Source: CAD feature listing. Evaluate the final solid. Frame: model axes, mm. A direction names the side the tool comes from. Give positions to 0.01 mm unless a question says otherwise; leave off trailing zeros. Order: outer loops, then holes, each group sorted by start corner. A loop starts at its lowest first (then second) coordinate and runs counter-clockwise, first axis right, second up. Notation, with made-up numbers: (33, -6) -> (68, -6) arc R16 ccw to (68, 12) -> close; hole circle Ø7 at (58.5, -32.5). An arc over 180 degrees is marked (long way). Answer in a Markdown table with one row per item.
```python
from build123d import *

# Parameters (mm, degrees)
BOSS_EXTRUDE1_DEPTH = 10
SKETCH4_R           = 2.5
BOSS_EXTRUDE3_DEPTH = 2.5


with BuildPart() as part:
    # Sketch1 → Boss-Extrude1 (new body)
    with BuildSketch(Plane(origin=(0, 0, 0), x_dir=(0, 0, -1), z_dir=(1, 0, 0))):
        Polygon((0, 9.55), (1.824674268, 6.809777075), (4.775, 8.270542606), (4.985102807, 4.985102807), (8.270542606, 4.775), (6.809777075, 1.824674268), (9.55, 0), (6.809777075, -1.824674268), (8.270542606, -4.775), (4.985102807, -4.985102807), (4.775, -8.270542606), (1.824674268, -6.809777075), (0, -9.55), (-1.824674268, -6.809777075), (-4.775, -8.270542606), (-4.985102807, -4.985102807), (-8.270542606, -4.775), (-6.809777075, -1.824674268), (-9.55, 0), (-6.809777075, 1.824674268), (-8.270542606, 4.775), (-4.985102807, 4.985102807), (-4.775, 8.270542606), (-1.824674268, 6.809777075), align=None)
    boss_extrude1 = extrude(amount=-BOSS_EXTRUDE1_DEPTH)

    # Sketch4 → Boss-Extrude3 (add)
    with BuildSketch(Plane(origin=(0, 0, 0), x_dir=(0, 0, -1), z_dir=(1, 0, 0))):
        Circle(SKETCH4_R)
    boss_extrude3 = extrude(amount=BOSS_EXTRUDE3_DEPTH)

    # Mirror1: Boss-Extrude1, Boss-Extrude3 across plane
    add(boss_extrude1.mirror(Plane.ZY.offset(10)))
    add(boss_extrude3.mirror(Plane.ZY.offset(10)))


solid = part.part
```
(1) Section query A-A (x = -16.75). Return the cut outline in (y, z) (3 decimals).
A:
| item | result |
|---|---|
| outline | (-9.55, 0) -> (-6.81, -1.825) -> (-8.271, -4.775) -> (-4.985, -4.985) -> (-4.775, -8.271) -> (-1.825, -6.81) -> (0, -9.55) -> (1.825, -6.81) -> (4.775, -8.271) -> (4.985, -4.985) -> (8.271, -4.775) -> (6.81, -1.825) -> (9.55, 0) -> (6.81, 1.825) -> (8.271, 4.775) -> (4.985, 4.985) -> (4.775, 8.271) -> (1.825, 6.81) -> (0, 9.55) -> (-1.825, 6.81) -> (-4.775, 8.271) -> (-4.985, 4.985) -> (-8.271, 4.775) -> (-6.81, 1.825) -> close |
(2) Pull-direction query (Z, two-part tool) for faces 1 (the flat face through (-10.14, -7.55, -3.32)), 2 (the flat face through (-10.14, -3.28, -7.53)), 3 (the flat face through (-10.14, 6.6, 4.88)); classes: +Z half, -Z half, draft (parallel to the pull), parting line (faces both ways), or undercut.
A:
| item | result |
|---|---|
| face 1 | undercut |
| face 2 | -Z half |
| face 3 | +Z half |
(3) First-contact query: pin 1 Ø10 at (x, y) = (-6.5, 4.5) entering from -Z; pin 2 Ø3 at (x, y) = (-5.5, -5) entering from +Z; pin 3 Ø10 at (x, z) = (-2, -6) entering from -Y; pin 4 Ø5 at (y, z) = (7, 3) entering from +X. Flat tips, straight axial feed; report the tip coordinate or a pass-through.
A:
| item | result |
|---|---|
| pin 1 | stops at z = -9.55 |
| pin 2 | stops at z = 8.27 |
| pin 3 | stops at y = -8.27 |
| pin 4 | stops at x = 0 |
(4) Section query B-B (z = 1.5). Return the cut outline in (x, y).
A:
| item | result |
|---|---|
| outline | (-22.5, -2) -> (-20, -2) -> (-20, -7.3) -> (0, -7.3) -> (0, -2) -> (2.5, -2) -> (2.5, 2) -> (0, 2) -> (0, 7.3) -> (-20, 7.3) -> (-20, 2) -> (-22.5, 2) -> close |
(5) Section query D-D (z = 4.25). Return the cut outline in (x, y).
A:
| item | result |
|---|---|
| outline | (-20, -8.01) -> (0, -8.01) -> (0, 8.01) -> (-20, 8.01) -> close |
(6) Access query for faces 4 (the flat face through (-10.14, -7.53, 3.28)), 5 (the cylindrical face through (1.23, -2.44, 0.54)), 6 (the cylindrical face through (-21.23, -2.44, 0.54)), 7 (the flat face through (-10.1, 8.2, -0.9)), 8 (the flat face through (-10.1, 0.9, -8.2)). Directions: +Z, -Z, +X, -X, +Y, -Y. A direction counts if a zero-diameter tool reaches every point of the face in a straight line with its end or side. Return the directions, or none.
A:
| item | result |
|---|---|
| face 4 | +X, -X, -Y |
| face 5 | +X |
| face 6 | -X |
| face 7 | +X, -X, +Y |
| face 8 | -Z, +X, -X |
(7) Ray query, probe 1 along Z at (x, y) = (-11, -7.5); probe 2 along Z at (x, y) = (-4.25, -7.25); probe 3 along Y at (x, z) = (-3.5, -7.75). Return the intervals inside material, ascending.
A:
| item | result |
|---|---|
| probe 1 | z = -4.82 to -3.22, -1.37 to 1.37, 3.22 to 4.82 |
| probe 2 | z = -4.84 to -2.71, -1.53 to 1.53, 2.71 to 4.84 |
| probe 3 | y = -4.81 to -3.72, -1.2 to 1.2, 3.72 to 4.81 |
